Part model, mm, in its own coordinate system. Face numbers are marked on the shaded views. A direction names the side the tool comes from. Give positions to 0.01 mm unless a question says otherwise; leave off trailing zeros. Loops run counter-clockwise (first coordinate to the right, second up) from the corner with the lowest first, then second, coordinate; pieces in that order, holes last. Notation, with made-up numbers: M 52,43 L 93,43 A20 cw 93,73 Z; hole C 88,-14.5 d6. An arc over 180 degrees is marked long. Answer in a Markdown table with one row per item.
from build123d import *

# Parameters (mm, degrees)
SKETCH1_W                   = 162
SKETCH1_H                   = 82
BOSS_EXTRUDE1_DEPTH         = 13
SKETCH2_W                   = 54
SKETCH2_H                   = 3
CUT_EXTRUDE1_DEPTH          = 83
SKETCH3_W                   = 54
SKETCH3_H                   = 3
CUT_EXTRUDE2_DEPTH          = 83
SKETCH4_W                   = 46
SKETCH4_H                   = 3
CUT_EXTRUDE3_DEPTH          = 83
SKETCH5_W                   = 14
SKETCH5_H                   = 58
CUT_EXTRUDE4_DEPTH          = 11
SKETCH6_W                   = 14
SKETCH6_H                   = 58
CUT_EXTRUDE5_DEPTH          = 14
F_3_8_CLEARANCE_HOLE1_D     = 10
F_3_8_CLEARANCE_HOLE1_DEPTH = 10
FILLET1_R                   = 2


with BuildPart() as part:
    # Sketch1 → Boss-Extrude1 (new body)
    with BuildSketch(Plane(origin=(0, 8, 0), x_dir=(1, 0, 0), z_dir=(0, 1, 0))):
        Rectangle(SKETCH1_W, SKETCH1_H)
    extrude(amount=-BOSS_EXTRUDE1_DEPTH)

    # Sketch2 → Cut-Extrude1 (cut, through all)
    with BuildSketch(Plane(origin=(0, 0, -41), x_dir=(-1, 0, 0), z_dir=(0, 0, -1))):
        with Locations((-54, 6.5)):
            Rectangle(SKETCH2_W, SKETCH2_H)
    extrude(amount=-CUT_EXTRUDE1_DEPTH, mode=Mode.SUBTRACT)

    # Sketch3 → Cut-Extrude2 (cut, through all)
    with BuildSketch(Plane(origin=(0, 0, -41), x_dir=(-1, 0, 0), z_dir=(0, 0, -1))):
        with Locations((54, 6.5)):
            Rectangle(SKETCH3_W, SKETCH3_H)
    extrude(amount=-CUT_EXTRUDE2_DEPTH, mode=Mode.SUBTRACT)

    # Sketch4 → Cut-Extrude3 (cut, through all)
    with BuildSketch(Plane(origin=(0, 0, -41), x_dir=(-1, 0, 0), z_dir=(0, 0, -1))):
        with Locations((0, -3.5)):
            Rectangle(SKETCH4_W, SKETCH4_H)
    extrude(amount=-CUT_EXTRUDE3_DEPTH, mode=Mode.SUBTRACT)

    # Sketch5 → Cut-Extrude4 (cut, through all)
    with BuildSketch(Plane.XZ.offset(2)):
        with Locations((-10, 0)):
            Rectangle(SKETCH5_W, SKETCH5_H)
    extrude(amount=-CUT_EXTRUDE4_DEPTH, mode=Mode.SUBTRACT)

    # Sketch6 → Cut-Extrude5 (cut, through all)
    with BuildSketch(Plane(origin=(0, 8, 0), x_dir=(-1, 0, 0), z_dir=(0, 1, 0))):
        with Locations((-10, 0)):
            Rectangle(SKETCH6_W, SKETCH6_H)
    extrude(amount=-CUT_EXTRUDE5_DEPTH, mode=Mode.SUBTRACT)

    # 3/8 Clearance Hole1
    with Locations(Plane(origin=(0, 5, 0), x_dir=(1, 0, 0), z_dir=(0, 1, 0))):
        with Locations((-61, 27), (61, 27), (-61, -27), (61, -27)):
            Hole(F_3_8_CLEARANCE_HOLE1_D / 2, depth=F_3_8_CLEARANCE_HOLE1_DEPTH)

    # Fillet1
    fillet1_edges = [part.edges().sort_by_distance(p)[0] for p in [
        (-3, 3, 29),
        (-3, 3, -29),
        (-17, 3, -29),
        (-17, 3, 29),
        (3, 3, -29),
        (81, 0, 41),
        (17, 3, -29),
        (17, 3, 29),
        (3, 3, 29),
        (-81, 0, 41),
        (-81, 0, -41),
        (81, 0, -41),
    ]]
    fillet(fillet1_edges, radius=FILLET1_R)


solid = part.part
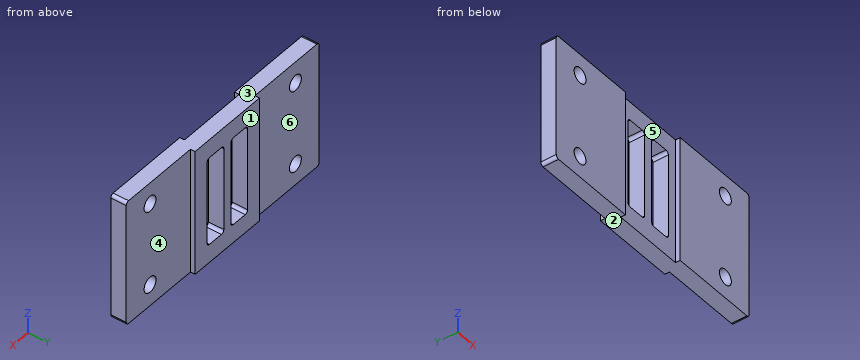
(1) Drill centre lines: line 1 along X through (y, z) = (0.25, -27); line 2 along Z through (x, y) = (61, 1); line 3 along X through (y, z) = (0, 11). Where is each one in solid material? Low to high.
Recorded:
| item | result |
|---|---|
| line 1 | x = -81 to -66, -56 to -17, -3 to 3, 17 to 56, 66 to 81 |
| line 2 | z = -41 to -32, -22 to 22, 32 to 41 |
| line 3 | x = -81 to -17, -3 to 3, 17 to 81 |
(2) Saw through at A-A (x = 61). Write the cut outline in (y, z).
Recorded:
| item | result |
|---|---|
| outline | M -5,-41 L 5,-41 L 5,-32 L -5,-32 Z; M -5,-22 L 5,-22 L 5,22 L -5,22 Z; M -5,32 L 5,32 L 5,41 L -5,41 Z |
(3) Saw through at C-C (x = -12). Write the cut outline in (y, z), plus the area to 3 significant figures.
Recorded:
| item | result |
|---|---|
| outline | M -2,-41 L 8,-41 L 8,-29 L -2,-29 Z; M -2,29 L 8,29 L 8,41 L -2,41 Z |
| area | 240 mm^2 |
(4) Which spindle directions (+Z, -Z, +X, -X, +Y, -Y) get a long thin tool onto all of the face, cutting with end or side? Do the marked faces 4, 5 and 6. Say none if no direction does.
Recorded:
| item | result |
|---|---|
| face 4 | +Z, -Z, +X, +Y |
| face 5 | +Z, -Z, -Y |
| face 6 | +Z, -Z, -X, +Y |
(5) Pull direction Z, two halves, no side cores. Call the marked faces 1, 2 and 3: +Z half, -Z half, draft (parallel to the pull), parting line (faces both ways), or undercut.
Recorded:
| item | result |
|---|---|
| face 1 | draft |
| face 2 | -Z half |
| face 3 | +Z half |
(6) Saw through at B-B (y = 1). Write the cut outline in (x, z), plus the area to 3 significant figures.
Recorded:
| item | result |
|---|---|
| outline | M -81,-39 A2 ccw -79,-41 L 79,-41 A2 ccw 81,-39 L 81,39 A2 ccw 79,41 L -79,41 A2 ccw -81,39 Z; hole C -61,-27 d10; hole C -61,27 d10; hole M -17,-27 A2 ccw -15,-29 L -5,-29 A2 ccw -3,-27 L -3,27 A2 ccw -5,29 L -15,29 A2 ccw -17,27 Z; hole M 3,-27 A2 ccw 5,-29 L 15,-29 A2 ccw 17,-27 L 17,27 A2 ccw 15,29 L 5,29 A2 ccw 3,27 Z; hole C 61,-27 d10; hole C 61,27 d10 |
| area | 11,300 mm^2 |
(7) Pin check, flat tips, straight feed: pin 1 Ø13 at (x, z) = (-61, 27) entering from +Y; pin 2 Ø2 at (y, z) = (6.5, 21.5) entering from +X. Stop position of each tip, or through.
Recorded:
| item | result |
|---|---|
| pin 1 | stops at y = 5 |
| pin 2 | stops at x = 27 |
